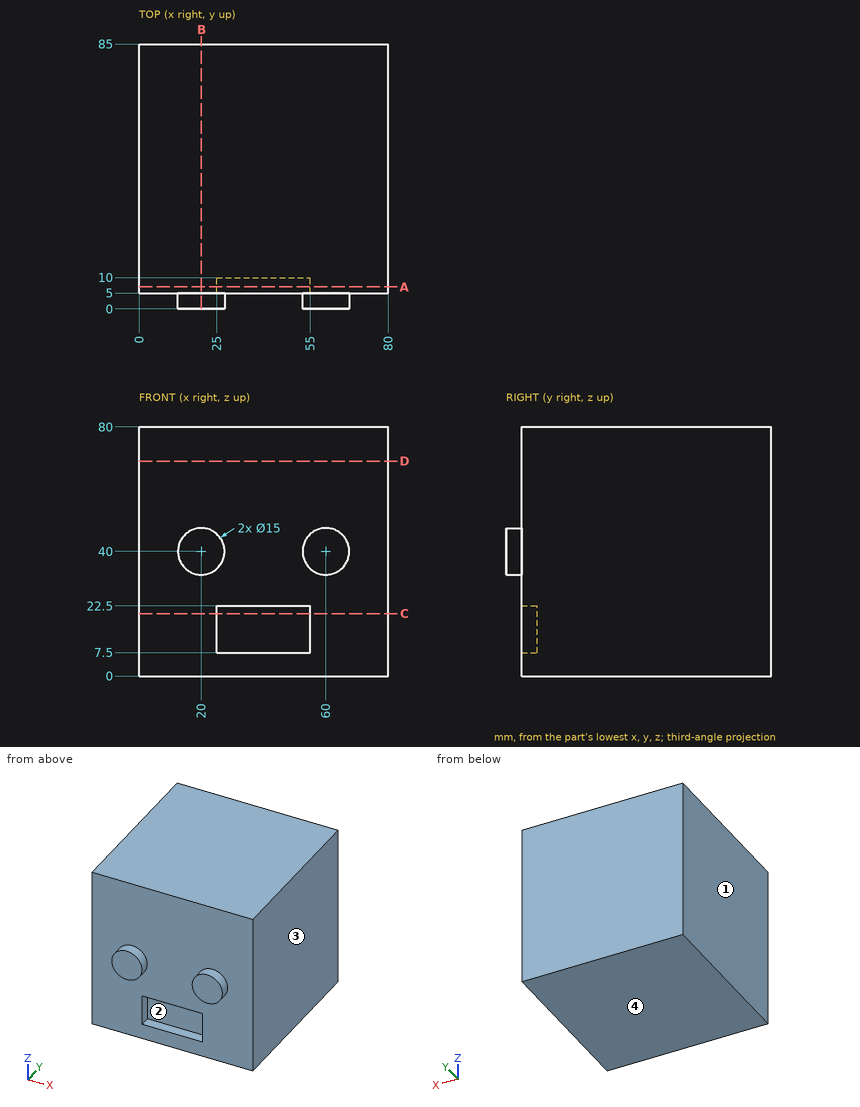
Part print with two shaded views. Sizes in mm from the minimum x, y, z corner. Round coordinates to 2 decimals unless told otherwise and drop trailing zeros. Order: outer loops, then holes, each group sorted by start corner. A loop starts at its lowest first (then second) coordinate and runs counter-clockwise, first axis right, second up. Notation, with made-up numbers: M 47.25,23 L 104.25,23 A26 ccw 104.25,48 Z; hole C -31,-37.5 d10. An arc over 180 degrees is marked long. Use CSV: the item, a comma, the result in double quotes. Start each with the question number.
(1) Drill centre lines: probe 1 along Y at (x, z) = (33, 54.5); probe 2 along X at (y, z) = (8, 15). Where is each one in solid material? Low to high.
(2) Cut at D-D on z = 69. List the corners of the cut face in (x, y), then the cut area to 3 significant figures.
(3) Cut at B-B on x = 20. List the corners of the cut face in (y, z).
(4) Cut at C-C on z = 20. List the corners of the cut face in (x, y).
(5) Mould opens along X. For the marked faces 1, 2, 3 and 4 say: +X half, -X half, draft (parallel to the pull), parting line (faces both ways), or undercut.
(6) Flat gauge pins, fed straight in: P1, Ø8, axis at y = 21, z = 27, coming from the -X side; P2, Ø16.5, axis at x = 36.5, z = 15.5, coming from the -Y side. Where does each tip first touch, or does it go through?
(7) Cut at A-A on y = 7. List the corners of the cut face in (x, z).
Findings:
1,probe 1,"y = 5 to 85"
1,probe 2,"x = 0 to 25, 55 to 80"
2,outline,"M 0,5 L 80,5 L 80,85 L 0,85 Z"
2,area,"6,400 mm^2"
3,outline,"M 0,32.5 L 5,32.5 L 5,0 L 85,0 L 85,80 L 5,80 L 5,47.5 L 0,47.5 Z"
4,outline,"M 0,5 L 25,5 L 25,10 L 55,10 L 55,5 L 80,5 L 80,85 L 0,85 Z"
5,face 1,"-X half"
5,face 2,"undercut"
5,face 3,"+X half"
5,face 4,"draft"
6,P1,"stops at x = 0"
6,P2,"stops at y = 5"
7,outline,"M 0,0 L 80,0 L 80,80 L 0,80 Z; hole M 25,7.5 L 55,7.5 L 55,22.5 L 25,22.5 Z"
